Study the drawing (mm; zero at the part's minimum x, y, z) and answer. Coordinates: 2 decimals unless noted, no trailing zeros. Write each loop counter-clockwise with the first axis right and the second up, starting at its lowest first coordinate (ties: lowest second). Pieces come first, ordered by that corner, then holes. Notation, with made-up numbers: M 73.5,14 L 79.5,14 A26 cw 79.5,41 Z; hole C -11,63.25 d11. An arc over 180 degrees is marked long. Answer as CSV lines item,"result". Start each with the question number.
(1) Find the intervals of material crossed by L1, parallel to X at y = 1.85, z = 7.5; L2, parallel to X at y = 0.7, z = 12.5; L3, parallel to Z at x = 6.25, y = 7 (1 decimal), in increasing order. Write a range as [from, to].
(2) A cutting plane is placed at A-A on z = 7.5. Give the vertices of the cut face in (x, y) (3 decimals), then the cut area to 3 significant figures.
(3) A cutting plane is placed at B-B on x = 7.5. Give the vertices of the cut face in (y, z) (3 decimals).
(4) A cutting plane is placed at C-C on y = 17.5. Give the vertices of the cut face in (x, z).
(5) A cutting plane is placed at D-D on y = 13. Give the vertices of the cut face in (x, z).
(6) The mould has two halves that part along Z. Classify the marked faces 1, 2, 3 and 4: released by +Z, released by -Z, zero draft, split by the parting line, or undercut.
(7) Flat-ended cylindrical pins translate along their axes: P1, Ø1, axis at x = 3, y = 11, coming from the +Z side; P2, Ø6, axis at x = 12.5, y = 5.5, coming from the -Z side; P3, Ø3, axis at y = 8, z = 11, coming from the +X side. Find the tip coordinate at first contact, or state that the pin passes through.
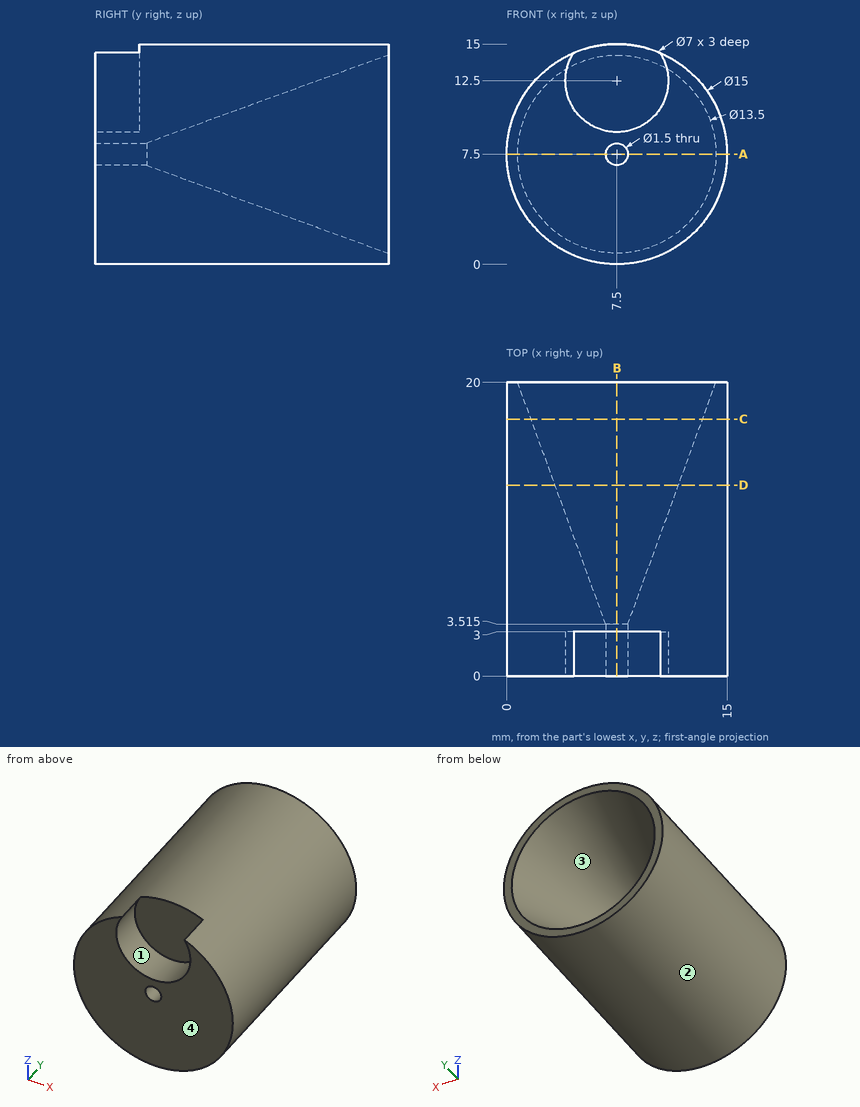
Here are the results:
1,L1,"x = [0, 6.75], [8.25, 15]"
1,L2,"x = [1.91, 4], [11, 13.09]"
1,L3,"z = [0.1, 5.9], [9.1, 14.9]"
2,outline,"M 0,0 L 6.75,0 L 6.75,3.515 L 0.75,20 L 0,20 Z; M 8.25,0 L 15,0 L 15,20 L 14.25,20 L 8.25,3.515 Z"
2,area,"171 mm^2"
3,outline,"M 0,0 L 20,0 L 20,0.75 L 3.515,6.75 L 0,6.75 Z; M 0,8.25 L 3.515,8.25 L 20,14.25 L 20,15 L 3,15 L 3,9 L 0,9 Z"
4,outline,"C 7.5,7.5 d15; hole C 7.5,7.5 d11.68"
5,outline,"C 7.5,7.5 d15; hole C 7.5,7.5 d8.4"
6,face 1,"undercut"
6,face 2,"split by the parting line"
6,face 3,"undercut"
6,face 4,"zero draft"
7,P1,"stops at z = 13.84"
7,P2,"stops at z = 0.27"
7,P3,"stops at x = 14.73"
